Autodesk Inventor part; units mm, degrees
ref_plane "YZ Plane" through (0, 0, 0) normal (1, 0, 0) x (0, 1, 0)
ref_plane "XZ Plane" through (0, 0, 0) normal (0, 1, 0) x (-1, 0, 0)
ref_plane "XY Plane" through (0, 0, 0) normal (0, 0, 1) x (1, 0, 0)
sketch "Sketch1" plane through (0, 0, 0) normal (0, 0, 1) x (1, 0, 0)
  circle A0 centre (0, 0) radius 5.4
  dimension "d0" = 10.8
extrude "Extrusion1" add sketch "Sketch1" against normal blind 17.9
sketch "Sketch2" plane through (0, 0, 0) normal (0, 0, 1) x (1, 0, 0)
  line L0 (3.4641, 6) -> (6.9282, 0)
  line L1 (6.9282, 0) -> (3.4641, -6)
  line L2 (3.4641, -6) -> (-3.4641, -6)
  line L3 (-3.4641, -6) -> (-6.9282, 0)
  line L4 (-6.9282, 0) -> (-3.4641, 6)
  line L5 (-3.4641, 6) -> (3.4641, 6)
  point P0 (0, 0)
  point P1 (0, 0)
  dimension "d4" = 12
extrude "Extrusion2" add sketch "Sketch2" against normal blind 5.8
sketch "Sketch3" plane through (0, 0, 0) normal (0, 0, 1) x (1, 0, 0)
  circle A0 centre (0, 0) radius 2
  dimension "d7" = 4
extrude "Extrusion3" cut sketch "Sketch3" against normal through all
properties part number "pin motor"
Part model, mm, in its own coordinate system. A direction names the side the tool comes from. Give positions to 0.01 mm unless a question says otherwise; leave off trailing zeros. Loops run counter-clockwise (first coordinate to the right, second up) from the corner with the lowest first, then second, coordinate; pieces in that order, holes last. Notation, with made-up numbers: M -39.5,23.5 L 17.5,23.5 A24 cw 17.5,58.5 Z; hole C -8.75,-32 d3. An arc over 180 degrees is marked long. Put each result on its own line as item: value. Start each with the question number.
1) Saw through at D-D (y = -3). List the corners of the cut face in (x, z).
2) Probe probe 1 along Y at (x, z) = (0, -8); probe 2 along Y at (x, z) = (0, -5.5); probe 3 along Z at (x, y) = (-4.5, 4). List the from-to ranges inside material, lowest first.
3) Saw through at A-A (x = 0). List the corners of the cut face in (y, z), then the cut area to 3 significant figures.
4) Saw through at C-C (z = -11). List the corners of the cut face in (x, y), then the cut area to 3 significant figures.
5) Flat gauge pins, fed straight in: pin 1 (4 mm diameter, centred on x = 3, y = -5, fed in from +Z); pin 2 (1.5 mm diameter, centred on x = -5, z = -13.5, fed in from +Y). Where does each tip first touch, or does it go through?
6) Saw through at B-B (y = 0.5). List the corners of the cut face in (x, z), then the cut area to 3 significant figures.
7) 3-axis set-ups, long thin cutter, end or side, ignore diameter. For faces 1 (the flat face through (4, 4, -5.8)), 2 (the flat face through (-5.22, 2.96, -2.86)): which of +Z, -Z, +X, -X, +Y, -Y reach the whole face in a straight line?
Numbers:
1. outline: M -5.2,-5.8 L -4.49,-5.8 L -4.49,-17.9 L 4.49,-17.9 L 4.49,-5.8 L 5.2,-5.8 L 5.2,0 L -5.2,0 Z
2. probe 1: -5.4 to -2, 2 to 5.4
2. probe 2: -6 to -2, 2 to 6
2. probe 3: -5.8 to 0
3. outline: M -6,-5.8 L -5.4,-5.8 L -5.4,-17.9 L -2,-17.9 L -2,0 L -6,0 Z; M 2,-17.9 L 5.4,-17.9 L 5.4,-5.8 L 6,-5.8 L 6,0 L 2,0 Z
3. area: 129 mm^2
4. outline: C 0,0 d10.8; hole C 0,0 d4
4. area: 79.0 mm^2
5. pin 1: z = 0
5. pin 2: y = 3.33
6. outline: M -6.64,-5.8 L -5.38,-5.8 L -5.38,-17.9 L -1.94,-17.9 L -1.94,0 L -6.64,0 Z; M 1.94,-17.9 L 5.38,-17.9 L 5.38,-5.8 L 6.64,-5.8 L 6.64,0 L 1.94,0 Z
6. area: 138 mm^2
7. face 1: -Z
7. face 2: +Z, -Z, -X, +Y
